Can you work these out from the model? Positions are in its coordinate system, mm. A direction names the side the tool comes from. Round coordinates to 2 decimals unless told otherwise and drop trailing zeros. Loops run counter-clockwise (first coordinate to the right, second up) from the corner with the lowest first, then second, coordinate; pieces in that order, holes last. Notation, with made-up numbers: M 57.5,11 L 98.5,11 A30 cw 98.5,48 Z; hole C -38.75,68.25 d2. An arc over 180 degrees is marked long. Return JSON: item names as keys, results as strings.
Autodesk Inventor part; units mm, degrees
ref_plane "Work Plane1" through (25.5, 0, 5) normal (-1, 0, 0) x (0, 1, 0)
ref_plane "Work Plane2" through (0, 117.5, 5) normal (0, 1, 0) x (1, 0, 0)
ref_plane "YZ Plane" through (0, 0, 0) normal (1, 0, 0) x (0, 1, 0)
sketch "Sketch1" plane through (0, 0, 0) normal (0, 0, 1) x (1, 0, 0)
  line L0 (0, 0) -> (51, 0)
  line L1 (51, 0) -> (51, 235)
  line L2 (51, 235) -> (0, 235)
  line L3 (0, 235) -> (0, 0)
  dimension "d0" = 51
  dimension "d1" = 235
extrude "Extrusion1" add sketch "Sketch1" along normal blind 5
sketch "Sketch3" plane through (0, 0, 5) normal (0, 0, 1) x (1, 0, 0)
  line L0 (0, 0) -> (51, 0)
  line L1 (25.5, 0) -> (25.5, 235)
  line L2 (51, 235) -> (0, 235)
  line L3 (0, 235) -> (0, 0)
  line L4 (0, 117.5) -> (51, 117.5)
  line L5 (51, 0) -> (51, 235)
ref_plane "Work Plane1" through (25.5, 0, 5) normal (-1, 0, 0) x (0, 1, 0)
ref_plane "Work Plane2" through (0, 117.5, 5) normal (0, 1, 0) x (1, 0, 0)
sketch "Sketch4" plane through (0, 0, 5) normal (0, 0, 1) x (1, 0, 0)
  circle A0 centre (5.625, 29.5) radius 2.1
  circle A1 centre (16.875, 19.5) radius 2.1
  circle A2 centre (45.375, 29.5) radius 2.1
  circle A3 centre (34.125, 19.5) radius 2.1
  circle A4 centre (5.625, 205.5) radius 2.1
  circle A5 centre (45.375, 205.5) radius 2.1
  circle A6 centre (34.125, 215.5) radius 2.1
  circle A7 centre (16.875, 215.5) radius 2.1
  point P0 (0, 0)
  dimension "d10" = 4.2
  dimension "d11" = 4.2
  dimension "d12" = 4.2
  dimension "d13" = 4.2
  dimension "d14" = 4.2
  dimension "d15" = 4.2
  dimension "d16" = 4.2
  dimension "d17" = 4.2
sketch "Sketch8" plane through (0, 0, 5) normal (0, 0, 1) x (1, 0, 0)
  line L0 (0, 0) -> (51, 0)
  line L1 (25.5, 0) -> (25.5, 235)
  line L2 (51, 235) -> (0, 235)
  line L3 (0, 235) -> (0, 0)
  line L4 (0, 117.5) -> (51, 117.5)
  line L5 (51, 0) -> (51, 235)
  line L6 (43.5, 99.5) -> (7.5, 99.5)
  line L7 (7.5, 99.5) -> (7.5, 135.5)
  line L8 (7.5, 135.5) -> (43.5, 135.5)
  line L9 (43.5, 135.5) -> (43.5, 99.5)
  line L10 (43.5, 99.5) -> (7.5, 135.5) construction
  line L11 (7.5, 99.5) -> (43.5, 135.5) construction
  line L12 (40.75, 102.25) -> (10.25, 102.25)
  line L13 (10.25, 102.25) -> (10.25, 132.75)
  line L14 (10.25, 132.75) -> (40.75, 132.75)
  line L15 (40.75, 132.75) -> (40.75, 102.25)
  line L16 (40.75, 102.25) -> (10.25, 132.75) construction
  line L17 (10.25, 102.25) -> (40.75, 132.75) construction
  line L18 (13, 105) -> (7.5, 105)
  line L19 (7.5, 105) -> (7.5, 99.5)
  line L20 (7.5, 99.5) -> (13, 99.5)
  line L21 (13, 99.5) -> (13, 105)
  line L22 (13, 105) -> (7.5, 99.5) construction
  line L23 (7.5, 105) -> (13, 99.5) construction
  line L24 (13, 130) -> (7.5, 130)
  line L25 (7.5, 130) -> (7.5, 135.5)
  line L26 (7.5, 135.5) -> (13, 135.5)
  line L27 (13, 135.5) -> (13, 130)
  line L28 (13, 130) -> (7.5, 135.5) construction
  line L29 (7.5, 130) -> (13, 135.5) construction
  line L30 (38, 105) -> (43.5, 105)
  line L31 (43.5, 105) -> (43.5, 99.5)
  line L32 (43.5, 99.5) -> (38, 99.5)
  line L33 (38, 99.5) -> (38, 105)
  line L34 (38, 105) -> (43.5, 99.5) construction
  line L35 (43.5, 105) -> (38, 99.5) construction
  line L36 (38, 130) -> (43.5, 130)
  line L37 (43.5, 130) -> (43.5, 135.5)
  line L38 (43.5, 135.5) -> (38, 135.5)
  line L39 (38, 135.5) -> (38, 130)
  line L40 (38, 130) -> (43.5, 135.5) construction
  line L41 (43.5, 130) -> (38, 135.5) construction
  point P0 (25.5, 117.5)
  dimension "d36" = 36
  dimension "d37" = 36
  dimension "d38" = 30.5
  dimension "d39" = 30.5
extrude "Extrusion8" add sketch "Sketch8" along normal blind 5 contours L33 L12 L15 L30 L9 L6 | L6 L7 L18 L13 L12 L21 | L7 L8 L27 L14 L13 L24 | L33 L30 L15 L12 | L12 L13 L18 L21 | L13 L14 L27 L24 | L36 L15 L14 L39 L8 L9 | L36 L39 L14 L15
sketch "Sketch9" plane through (0, 0, 10) normal (0, 0, 1) x (1, 0, 0)
  line L0 (7.5, 99.5) -> (13, 99.5)
  line L1 (10.25, 99.5) -> (10.25, 105)
  line L2 (13, 105) -> (7.5, 105)
  line L3 (13, 99.5) -> (13, 105)
  line L4 (13, 102.25) -> (7.5, 102.25)
  line L5 (7.5, 99.5) -> (7.5, 105)
  point P0 (0, 0)
  point P1 (10.25, 102.25)
hole "Hole1" at (10.25, 102.25, 10) direction (0, 0, -1) diameter 2.616 depth 5
sketch "Sketch10" plane through (0, 0, 5) normal (0, 0, 1) x (1, 0, 0)
  line L0 (0, 0) -> (51, 0)
  line L1 (25.5, 0) -> (25.5, 235)
  line L2 (51, 235) -> (0, 235)
  line L3 (0, 235) -> (0, 0)
  line L4 (0, 117.5) -> (51, 117.5)
  line L5 (51, 0) -> (51, 235)
  point P0 (0, 185)
  point P1 (0, 50)
  point P2 (51, 50)
  point P3 (51, 185)
sketch "Sketch11" plane through (0, 0, 5) normal (0, 0, 1) x (1, 0, 0)
  point P0 (0, 0)
sketch "Sketch12" plane through (0, 0, 5) normal (0, 0, 1) x (1, 0, 0)
  line L0 (51, 50) -> (0, 50)
  line L1 (0, 185) -> (3, 185)
  line L2 (3, 185) -> (3, 50)
  line L3 (3, 50) -> (0, 50)
  line L4 (0, 50) -> (0, 185)
  line L5 (51, 185) -> (48, 185)
  line L6 (48, 185) -> (48, 50)
  line L7 (48, 50) -> (51, 50)
  line L8 (51, 50) -> (51, 185)
  point P0 (0, 0)
  dimension "d51" = 3
  dimension "d52" = 3
extrude "Extrusion9" add sketch "Sketch12" along normal blind 4
mirror "Mirror5" about plane through (25.5, 0, 5) normal (-1, 0, 0) of "Hole1"
mirror "Mirror6" about plane through (0, 117.5, 5) normal (0, 1, 0) of "Hole1", "Mirror5"
sketch "Sketch15" plane through (0, 0, 5) normal (0, 0, 1) x (1, 0, 0)
  circle A0 centre (45.375, 29.5) radius 4.25
  circle A1 centre (34.125, 19.5) radius 4.25
  circle A2 centre (16.875, 19.5) radius 4.25
  circle A3 centre (5.625, 29.5) radius 4.25
  circle A4 centre (5.625, 205.5) radius 4.25
  circle A5 centre (16.875, 215.5) radius 4.25
  circle A6 centre (34.125, 215.5) radius 4.25
  circle A7 centre (45.375, 205.5) radius 4.25
  line L0 (51, 0) -> (51, 50)
  line L1 (0, 0) -> (51, 0)
  circle A8 centre (45.375, 29.5) radius 2.1
  circle A9 centre (34.125, 19.5) radius 2.1
  line L2 (0, 50) -> (0, 0)
  line L3 (0, 235) -> (0, 185)
  line L4 (51, 235) -> (0, 235)
  line L5 (51, 185) -> (51, 235)
  circle A10 centre (5.625, 205.5) radius 2.1
  circle A11 centre (16.875, 215.5) radius 2.1
  circle A12 centre (34.125, 215.5) radius 2.1
  circle A13 centre (45.375, 205.5) radius 2.1
  line L6 (0, 0) -> (51, 0)
  line L7 (51, 50) -> (0, 50)
  line L8 (0, 235) -> (51, 235)
  line L9 (51, 185) -> (0, 185)
  arc A14 (51, 24.5392) -> (51, 34.4608) centre (45.375, 29.5) ccw
  arc A15 (0, 34.4608) -> (0, 24.5392) centre (5.625, 29.5) ccw
  arc A16 (0, 210.4608) -> (0, 200.5392) centre (5.625, 205.5) ccw
  arc A17 (51, 200.5392) -> (51, 210.4608) centre (45.375, 205.5) ccw
  line L10 (0, 50) -> (0, 34.4608)
  line L11 (0, 24.5392) -> (0, 0)
  line L12 (51, 0) -> (51, 24.5392)
  line L13 (51, 34.4608) -> (51, 50)
  line L14 (0, 185) -> (0, 200.5392)
  line L15 (0, 210.4608) -> (0, 235)
  line L16 (51, 235) -> (51, 210.4608)
  line L17 (51, 200.5392) -> (51, 185)
  dimension "d78" = 8.5
  dimension "d79" = 8.5
  dimension "d80" = 8.5
  dimension "d81" = 8.5
  dimension "d82" = 8.5
  dimension "d83" = 8.5
  dimension "d84" = 8.5
  dimension "d85" = 8.5
  dimension "d86" = 5.625
  dimension "d87" = 29.5
  dimension "d88" = 19.5
  dimension "d89" = 16.875
  dimension "d90" = 4.2
  dimension "d91" = 4.2
  dimension "d92" = 19.5
  dimension "d93" = 16.875
  dimension "d94" = 5.625
  dimension "d95" = 29.5
  dimension "d96" = 5.625
  dimension "d97" = 29.5
  dimension "d98" = 19.5
  dimension "d99" = 16.875
  dimension "d100" = 19.5
  dimension "d101" = 16.875
  dimension "d102" = 5.625
  dimension "d103" = 29.5
  dimension "d104" = 4.2
  dimension "d105" = 4.2
  dimension "d106" = 4.2
  dimension "d107" = 4.2
  dimension "d108" = 15
  dimension "d109" = 15
  dimension "d110" = 15
  dimension "d111" = 15
extrude "Extrusion11" add sketch "Sketch15" along normal blind 4 contours L1 L2 L7 L0 | L0 A14 | A15 L2 | L4 L5 L9 L3 | L3 A16 | A17 L5
sketch "Sketch16" plane through (5.625, 29.5, 5) normal (0, 0, 1) x (1, 0, 0)
  circle A0 centre (11.25, -10) radius 2.1
  circle A1 centre (0, 0) radius 2.1
  circle A2 centre (28.5, -10) radius 2.1
  circle A3 centre (39.75, 0) radius 2.1
  circle A4 centre (39.75, 176) radius 2.1
  circle A5 centre (28.5, 186) radius 2.1
  circle A6 centre (11.25, 186) radius 2.1
  circle A7 centre (0, 176) radius 2.1
  line L0 (-5.625, -4.9608) -> (-5.625, -29.5)
  line L1 (-5.625, -29.5) -> (45.375, -29.5)
  line L2 (45.375, -29.5) -> (45.375, -4.9608)
  line L3 (45.375, 4.9608) -> (45.375, 20.5)
  line L4 (-5.625, 205.5) -> (-5.625, 180.9608)
  line L5 (45.375, 205.5) -> (-5.625, 205.5)
  line L6 (45.375, 180.9608) -> (45.375, 205.5)
  dimension "d115" = 4.2
  dimension "d116" = 4.2
  dimension "d117" = 4.2
  dimension "d118" = 4.2
  dimension "d119" = 5.625
  dimension "d120" = 29.5
  dimension "d121" = 19.5
  dimension "d122" = 34.125
  dimension "d123" = 19.5
  dimension "d124" = 16.875
  dimension "d125" = 4.2
  dimension "d126" = 4.2
  dimension "d127" = 5.625
  dimension "d128" = 29.5
  dimension "d129" = 4.2
  dimension "d130" = 4.2
  dimension "d131" = 5.625
  dimension "d132" = 29.5
  dimension "d133" = 19.5
  dimension "d134" = 34.125
  dimension "d135" = 19.5
  dimension "d136" = 16.875
  dimension "d137" = 5.625
  dimension "d138" = 29.5
extrude "Extrusion12" cut sketch "Sketch16" against normal blind 5
ref_plane "Work Plane5" through (0, 235, 5) normal (0.7071, 0, -0.7071) x (0, -1, 0)
sketch "Sketch18" plane through (0, 235, 5) normal (0.7071, 0, -0.7071) x (0, -1, 0)
  ellipse E0 centre (29.5, -3.9775) end of major axis (37, -3.9775) minor radius 5.3033 (34.4608, 0) -> (24.5392, 0) ccw
  line L0 (34.4608, 0) -> (24.5392, 0)
  point P0 (235, 3.5355)
sketch "Sketch19" plane through (0, 0, 5) normal (0, 0, -1) x (-1, 0, 0)
  line L0 (0, 233) -> (0, 2)
  arc A0 (0, 200.5392) -> (0, 210.4608) centre (-5.625, 205.5) ccw
  arc A1 (0, 200.5392) -> (0, 210.4608) centre (-5.625, 205.5) ccw
  line L1 (0, 210.4608) -> (0, 200.5392)
  line L2 (0, 235) -> (0, 0)
revolve "Revolution1" add sketch "Sketch19" angle 90 about axis through (0, 233, 5) along (0, -1, 0)
mirror "Mirror7" about plane through (0, 117.5, 5) normal (0, 1, 0) of "Revolution1"
mirror "Mirror8" about plane through (25.5, 0, 5) normal (-1, 0, 0) of "Revolution1", "Mirror7"
sketch "Sketch20" plane through (0, 0, 5) normal (0, 0, 1) x (1, 0, 0)
  circle A0 centre (10.5, 72.5) radius 1.6
  circle A1 centre (39.5, 72.5) radius 1.6
  circle A2 centre (10.5, 162.5) radius 1.6
  circle A3 centre (39.5, 162.5) radius 1.6
  point P0 (0, 0)
extrude "Extrusion13" cut sketch "Sketch20" against normal blind 5
sketch "Sketch21" plane through (0, 0, 9) normal (0, 0, 1) x (1, 0, 0)
  circle A0 centre (5.2, 5.2) radius 2.1
  line L0 (0, 0) -> (51, 0)
  line L1 (0, 24.5392) -> (0, 0)
  line L2 (25.5, 0) -> (25.5, 235)
  line L3 (0, 117.5) -> (51, 117.5)
  circle A1 centre (45.8, 5.2) radius 2.1
  circle A2 centre (5.2, 229.8) radius 2.1
  circle A3 centre (45.8, 229.8) radius 2.1
  dimension "d150" = 4.2
  dimension "d153" = 5.2
  dimension "d154" = 5.2
extrude "Extrusion14" cut sketch "Sketch21" against normal blind 9
fillet "Fillet3" radius 2 4 edges at (0, 0, 4.5) (51, 0, 4.5) (0, 235, 4.5) (51, 235, 4.5)
properties part number "Component plate" material "ABS Plastic"
Q1. Suppose I cut it at D-D, the plane y = 29.5. State how many separate pieces and enclosed holes the cut face has, plus the area to 3 significant figures.
Results:
{"separate pieces": "3", "enclosed holes": "0", "area": "370 mm2"}
Q2. Suppose I cut it at C-C, the plane y = 112.5. Please give me the cut outline in (x, z), plus the area to 3 significant figures.
Results:
{"outline": "M 0,0 L 51,0 L 51,9 L 48,9 L 48,5 L 3,5 L 3,9 L 0,9 Z", "area": "279 mm2"}
Q3. Suppose I cut it at A-A, the plane y = 229.8. Please give me the cut outline in (x, z), plus the area to 3 significant figures.
Results:
{"outline": "M 0,0 L 3.1,0 L 3.1,9 L 0,9 Z; M 7.3,0 L 43.7,0 L 43.7,9 L 7.3,9 Z; M 47.9,0 L 51,0 L 51,9 L 47.9,9 Z", "area": "383 mm2"}
Q4. Thinking about a two-plate mould opening in X: for faces 1 (the flat face through (38, 133, 7)), 2 (the flat face through (51, 116, 4)), 3 (the flat face through (25, 119, 0)), which applies, pulls with the +X half, pulls with the -X half, needs draft (parallel to the pull), parting line crosses it, or undercut?
Results:
{"face 1": "undercut", "face 2": "pulls with the +X half", "face 3": "needs draft"}
Q5. On a 3-axis mill with a long thin cutter (end or side, diameter ignored), from which of +Z, -Z, +X, -X, +Y, -Y can I reach the whole of each face in a straight line? I mean faces 4 (the flat face through (43, 205, 5)), 5 (the cylindrical face through (52.875, 29.576, 6.972)). Say none if no direction works.
Results:
{"face 4": "+Z", "face 5": "+Z, -Z, +X"}
Q6. I'm going to push flat-ended pins straight in: pin 1 Ø13.5 at (x, y) = (33.5, 120) entering from +Z; pin 2 Ø5.5 at (y, z) = (101.5, 7.5) entering from -X; pin 3 Ø2 at (y, z) = (26.5, 4) entering from -X. Where does each tip first touch, or does it pass through?
Results:
{"pin 1": "stops at z = 5", "pin 2": "stops at x = 0", "pin 3": "stops at x = -1.49"}
Q7. Suppose I cut it at B-B, the plane x = 27.5. Please give me the cut outline in (y, z).
Results:
{"outline": "M 0,0 L 235,0 L 235,9 L 185,9 L 185,5 L 50,5 L 50,9 L 0,9 Z"}
Q8. If I drill on line 1 along X through (y, z) = (102.25, 6.1); line 2 along X through (y, z) = (205.5, 1.35) (3 decimals); line 3 along X through (y, z) = (229.8, 5.5), over which ranges is the centre line in solid material (lowest first)?
Results:
{"line 1": "x = 0 to 3, 7.5 to 8.94, 11.56 to 13, 38 to 39.44, 42.06 to 43.5, 48 to 51", "line 2": "x = 0 to 3.525, 7.725 to 43.275, 47.475 to 51", "line 3": "x = 0 to 3.1, 7.3 to 43.7, 47.9 to 51"}
